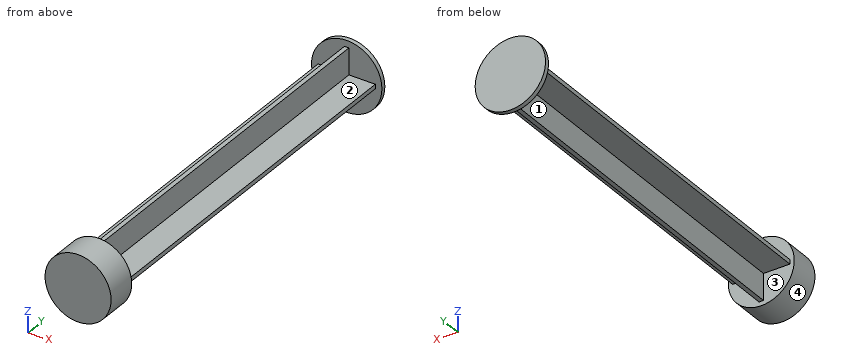
from build123d import *

# Parameters (mm, degrees)
F0_R     = 8
F1_DEPTH = 1
F2_W     = 6
F2_H     = 0.5
F2_W_2   = 0.5
F2_H_2   = 6
F3_DEPTH = 84
F4_R     = 7.5
F5_DEPTH = 7


with BuildPart() as f1:
    # F0 (on Front) → F1 (new body)
    with BuildSketch(Plane.XZ):
        Circle(F0_R)
    extrude(amount=F1_DEPTH)

    # F2 (on face) → F3 (join)
    with BuildSketch(Plane.XZ.offset(1)):
        with Locations((-3.5, 0.25)):
            Rectangle(F2_W, F2_H)
        with Locations((-3.5, -0.25)):
            Rectangle(F2_W, F2_H)
        with Locations((-0.25, 0.25)):
            Rectangle(F2_W_2, F2_H)
        with Locations((-0.25, -0.25)):
            Rectangle(F2_W_2, F2_H)
        with Locations((0.25, 0.25)):
            Rectangle(F2_W_2, F2_H)
        with Locations((0.25, -0.25)):
            Rectangle(F2_W_2, F2_H)
        with Locations((-0.25, -3.5)):
            Rectangle(F2_W_2, F2_H_2)
        with Locations((-0.25, 3.5)):
            Rectangle(F2_W_2, F2_H_2)
        with Locations((3.5, 0.25)):
            Rectangle(F2_W, F2_H)
        with Locations((3.5, -0.25)):
            Rectangle(F2_W, F2_H)
        with Locations((0.25, 3.5)):
            Rectangle(F2_W_2, F2_H_2)
        with Locations((0.25, -3.5)):
            Rectangle(F2_W_2, F2_H_2)
    extrude(amount=F3_DEPTH)

    # F4 (on face) → F5 (join)
    with BuildSketch(Plane.XZ.offset(85)):
        Circle(F4_R)
    extrude(amount=F5_DEPTH)


solid = f1.part
Work out the finished part from the listing and answer in its coordinate system (mm). Face numbers are marked on the shaded views. A direction names the side the tool comes from. Give positions to 0.01 mm unless a question says otherwise; leave off trailing zeros. Write each loop counter-clockwise with the first axis right and the second up, starting at its lowest first coordinate (ties: lowest second). Pieces come first, ordered by that corner, then holes. Notation, with made-up numbers: M 76,48.25 L 119,48.25 A15 ccw 119,74.25 Z; hole C 30,19 d3. An arc over 180 degrees is marked long. Answer as CSV lines item,"result".
Q1. Given P1, Ø0.5, axis at y = -26.5, z = 0, coming from the -X side; P2, Ø3, axis at x = 3.5, y = -33.5, coming from the -Z side; P3, Ø2, axis at x = -2.5, y = -32.5, coming from the +Z side, each flat-ended and moving along its own axis, determine where each tip first touches the part or whether it passes through.
A:
P1,"stops at x = -6.5"
P2,"stops at z = -0.5"
P3,"stops at z = 0.5"
Q2. A cutting plane is placed at A-A on y = -18.5. Write down the section's boundary in (x, z).
A:
outline,"M -6.5,-0.5 L -0.5,-0.5 L -0.5,-6.5 L 0.5,-6.5 L 0.5,-0.5 L 6.5,-0.5 L 6.5,0.5 L 0.5,0.5 L 0.5,6.5 L -0.5,6.5 L -0.5,0.5 L -6.5,0.5 Z"
Q3. A cutting plane is placed at B-B on x = -3.5. Write down the section's boundary in (y, z).
A:
outline,"M -92,-6.63 L -85,-6.63 L -85,-0.5 L -1,-0.5 L -1,-7.19 L 0,-7.19 L 0,7.19 L -1,7.19 L -1,0.5 L -85,0.5 L -85,6.63 L -92,6.63 Z"
Q4. A tool of negligible diameter and unlimited length cuts with its end or side. For the marked faces 1, 2, 3 and 4, from which of +Z, -Z, +X, -X, +Y, -Y can it reach the whole face along a straight path? Write none if from no direction.
A:
face 1,"-Z, -X"
face 2,"+Z, +X"
face 3,"none"
face 4,"-Y"
Q5. Find the intervals of material crossed by probe 1 along Y at (x, z) = (-2, 1.25); probe 2 along Z at (x, y) = (2, -54), in increasing order. Write a range as [from, to].
A:
probe 1,"y = [-92, -85], [-1, 0]"
probe 2,"z = [-0.5, 0.5]"
